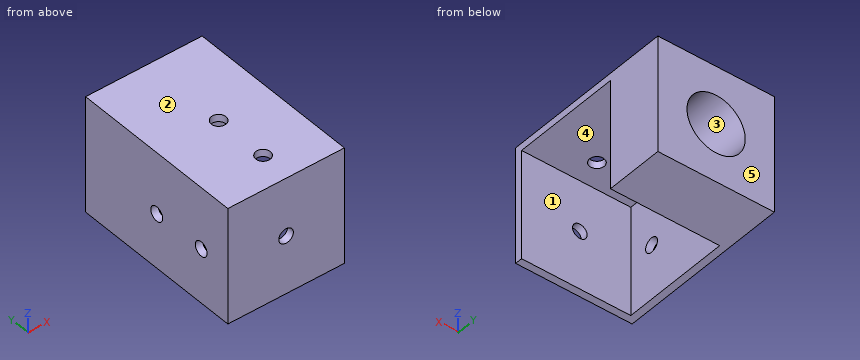
Autodesk Inventor part; units mm, degrees
ref_plane "YZ Plane" through (0, 0, 0) normal (1, 0, 0) x (0, 1, 0)
ref_plane "XZ Plane" through (0, 0, 0) normal (0, 1, 0) x (-1, 0, 0)
ref_plane "XY Plane" through (0, 0, 0) normal (0, 0, 1) x (1, 0, 0)
sketch "Sketch1" plane through (0, 0, 0) normal (0, 1, 0) x (-1, 0, 0)
  line L0 (0, 0) -> (50.8, 0)
  line L1 (50.8, 0) -> (50.8, -50.8)
  line L2 (50.8, -50.8) -> (0, -50.8)
  line L3 (0, -50.8) -> (0, 0)
  line L4 (47.625, -3.175) -> (3.175, -3.175)
  line L5 (3.175, -3.175) -> (3.175, -47.625)
  line L6 (3.175, -47.625) -> (47.625, -47.625)
  line L7 (47.625, -47.625) -> (47.625, -3.175)
  line L8 (47.625, -47.625) -> (47.625, -50.8)
  line L9 (3.175, -3.175) -> (0, -3.175)
  dimension "d0" = 50.8
  dimension "d1" = 50.8
  dimension "d2" = 3.175
extrude "Extrusion1" add sketch "Sketch1" against normal blind 25.4 contours L0 L1 L2 L8 L7 L4 L9 L3
sketch "Sketch2" plane through (0, 0, 0) normal (0, 1, 0) x (1, 0, 0)
  line L0 (-50.8, 0) -> (-50.8, 50.8)
  line L1 (-50.8, 0) -> (0, 0)
  line L2 (0, 0) -> (0, 50.8)
  line L3 (0, 50.8) -> (-50.8, 50.8)
  line L4 (-50.8, 50.8) -> (-50.8, 0)
  dimension "d5" = 50.8
extrude "Extrusion2" add sketch "Sketch2" along normal blind 25.4
sketch "Sketch3" plane through (0, 25.4, 0) normal (0, 1, 0) x (1, 0, 0)
  line L0 (-50.8, 0) -> (-50.8, 50.8) construction
  line L1 (-50.8, 0) -> (0, 50.8) construction
  line L2 (0, 0) -> (-50.8, 0) construction
  line L3 (0, 0) -> (-50.8, 50.8) construction
  point P0 (-25.61, 25.3161)
sketch "Sketch4" plane through (0, 25.4, 0) normal (0, 1, 0) x (1, 0, 0)
  point P0 (0, 0)
  point P1 (-25.3999, 25.4)
hole "Hole1" at (-25.3999, 25.4, -25.4) direction (0, -1, 0) diameter 25.4 end through all
sketch "Sketch5" plane through (0, -25.4, -3.175) normal (0, 0, -1) x (-1, 0, 0)
  line L0 (0, 25.4) -> (0, 0) construction
  line L1 (47.625, 0) -> (0, 0) construction
  line L2 (0, 25.4) -> (47.625, 0) construction
  line L3 (0, 25.4) -> (47.625, 25.4) construction
  line L4 (0, 0) -> (47.625, 25.4) construction
sketch "Sketch6" plane through (0, -25.4, -3.175) normal (0, 0, -1) x (-1, 0, 0)
  point P0 (0, 25.4)
  point P1 (23.8125, 12.7)
hole "Hole2" at (-23.8125, -12.7, -3.175) direction (0, 0, 1) diameter 6.35 end through all
sketch "Sketch7" plane through (-47.625, -25.4, -3.175) normal (1, 0, 0) x (0, 0, -1)
  line L0 (47.625, 0) -> (0, 0) construction
  line L1 (0, 25.4) -> (0, 0) construction
  line L2 (47.625, 0) -> (0, 25.4) construction
  line L3 (47.625, 25.4) -> (47.625, 0) construction
  line L4 (0, 0) -> (47.625, 25.4) construction
  point P0 (-3.175, 25.4)
sketch "Sketch8" plane through (-47.625, -25.4, -3.175) normal (1, 0, 0) x (0, 0, -1)
  point P0 (-3.175, 25.4)
  point P1 (23.8116, 12.6997)
hole "Hole3" at (-47.625, -12.7003, -26.9866) direction (-1, 0, 0) diameter 6.35 end through all
sketch "Sketch9" plane through (0, -25.4, 0) normal (0, -1, 0) x (1, 0, 0)
  line L0 (-50.8, -50.8) -> (-50.8, 0)
  line L1 (0, 0) -> (-50.8, 0)
  line L2 (-50.8, 0) -> (-50.8, -50.8)
  line L3 (-50.8, -50.8) -> (0, -50.8)
  line L4 (0, -50.8) -> (0, 0)
  line L5 (-47.625, -3.175) -> (-3.175, -3.175)
  line L6 (-3.175, -3.175) -> (-3.175, -47.625)
  line L7 (-3.175, -47.625) -> (-47.625, -47.625)
  line L8 (-47.625, -47.625) -> (-47.625, -3.175)
  line L9 (0, -3.175) -> (-47.625, -3.175)
  line L10 (-3.175, -3.175) -> (0, -3.175)
  line L11 (-47.625, -47.625) -> (-47.625, -50.8)
  point P0 (-3.175, -3.175)
extrude "Extrusion3" add sketch "Sketch9" along normal blind 25.4 contours L0 L1 L4 L9 L5 L8 L11 L3
sketch "Sketch10" plane through (0, -50.8, 0) normal (0, -1, 0) x (1, 0, 0)
  line L0 (0, 0) -> (-50.8, 0)
  line L1 (-50.8, 0) -> (-50.8, -50.8)
  line L2 (-50.8, -50.8) -> (0, -50.8)
  line L3 (0, -50.8) -> (0, 0)
extrude "Extrusion4" add sketch "Sketch10" against normal blind 3.175
sketch "Sketch11" plane through (0, 0, -3.175) normal (0, 0, -1) x (-1, 0, 0)
  line L0 (47.625, 0) -> (47.625, -47.625) construction
  line L1 (47.625, -47.625) -> (0, -25.4001) construction
  line L2 (0, 0) -> (0, -47.625) construction
  line L3 (0, -47.625) -> (47.625, -47.625) construction
  line L4 (47.625, -25.4001) -> (0, -47.625) construction
sketch "Sketch12" plane through (0, 0, -3.175) normal (0, 0, -1) x (-1, 0, 0)
  point P0 (0, 0)
  point P1 (23.8112, -36.5118)
hole "Hole4" at (-23.8112, -36.5118, -3.175) direction (0, 0, 1) diameter 6.35 end through all
sketch "Sketch13" plane through (-47.625, 0, -3.175) normal (1, 0, 0) x (0, 0, -1)
  line L0 (0, 0) -> (0, -47.625) construction
  line L1 (0, -47.625) -> (47.625, -47.625) construction
  line L2 (0, -25.4031) -> (47.625, -47.625) construction
  line L3 (0, -47.625) -> (47.625, -25.4031) construction
  line L4 (47.625, 0) -> (47.625, -47.625) construction
  point P0 (-3.175, 0)
sketch "Sketch14" plane through (-47.625, 0, -3.175) normal (1, 0, 0) x (0, 0, -1)
  point P0 (-3.175, 0)
  point P1 (23.8113, -36.5122)
hole "Hole5" at (-47.625, -36.5122, -26.9863) direction (-1, 0, 0) diameter 6.35 end through all
sketch "Sketch15" plane through (0, -47.625, 0) normal (0, 1, 0) x (1, 0, 0)
  line L0 (-50.8, 0) -> (-50.8, 50.8) construction
  line L1 (0, 0) -> (-50.8, 50.8) construction
  line L2 (0, 0) -> (0, 50.8) construction
  line L3 (-50.8, 0) -> (0, 50.8) construction
sketch "Sketch16" plane through (0, -47.625, 0) normal (0, 1, 0) x (1, 0, 0)
  point P0 (0, 0)
  point P1 (-25.4077, 25.4046)
hole "Hole6" at (-25.4077, -47.625, -25.4046) direction (0, -1, 0) diameter 6.35 end through all
properties part number "Bearing Housing"
The model under review builds one solid part; all positions refer to its coordinate system, in mm. Face numbers are marked on the shaded views. A direction names the side the tool comes from. Round coordinates to 2 decimals unless told otherwise and drop trailing zeros. Order: outer loops, then holes, each group sorted by start corner. A loop starts at its lowest first (then second) coordinate and runs counter-clockwise, first axis right, second up. Notation, with made-up numbers: M 50.5,69 L 68.5,69 A33 ccw 68.5,108 Z; hole C 58.5,-18.5 d10. An arc over 180 degrees is marked long. Use a Markdown table: item, result.
1) Consider section A-A (z = -27). Write out the cut boundary in (x, y) (3 decimals).
Report:
| item | result |
|---|---|
| outline | M -50.8,-50.8 L -28.153,-50.8 L -28.153,-47.625 L -47.625,-47.625 L -47.625,-39.687 L -50.8,-39.687 Z; M -50.8,-33.337 L -47.625,-33.337 L -47.625,-15.875 L -50.8,-15.875 Z; M -50.8,-9.525 L -47.625,-9.525 L -47.625,0 L -37.999,0 L -37.999,25.4 L -50.8,25.4 Z; M -22.663,-50.8 L 0,-50.8 L 0,-47.625 L -22.663,-47.625 Z; M -12.801,0 L 0,0 L 0,25.4 L -12.801,25.4 Z |
2) Consider section C-C (y = -11). Write out the cut boundary in (x, z) (3 decimals).
Report:
| item | result |
|---|---|
| outline | M -50.8,-50.8 L -47.625,-50.8 L -47.625,-29.668 L -50.8,-29.668 Z; M -50.8,-24.305 L -47.625,-24.305 L -47.625,-3.175 L -26.494,-3.175 L -26.494,0 L -50.8,0 Z; M -21.131,-3.175 L 0,-3.175 L 0,0 L -21.131,0 Z |
3) Wall thickness on line 1 along Y through (x, z) = (-30, -7) (3 decimals); line 2 along Z through (x, y) = (-26, 15.5); line 3 along Z through (x, y) = (-2.5, -22) (3 decimals): over which ranges is each line inside the solid? List them lowest first. Write a range as [from, to].
Report:
| item | result |
|---|---|
| line 1 | [-50.8, -47.625], [0, 25.4] |
| line 2 | [-50.8, -38.09], [-12.71, 0] |
| line 3 | [-3.175, 0] |
4) Consider section D-D (x = -34.5). Write out the cut boundary in (y, z) (3 decimals), then the cut area to 3 significant figures.
Report:
| item | result |
|---|---|
| outline | M -50.8,-50.8 L -47.625,-50.8 L -47.625,-3.175 L 0,-3.175 L 0,-16.541 L 25.4,-16.541 L 25.4,0 L -50.8,0 Z; M 0,-50.8 L 25.4,-50.8 L 25.4,-34.259 L 0,-34.259 Z |
| area | 1,150 mm^2 |
5) Draft analysis for pull direction Z (two halves, no side actions). For the marked faces 1, 2 and 3, state which applies: released by +Z, released by -Z, zero draft, split by the parting line, or undercut.
Report:
| item | result |
|---|---|
| face 1 | zero draft |
| face 2 | released by +Z |
| face 3 | undercut |
6) Insertion check: pin 1 (1 mm diameter, centred on x = -9, y = -9.5, fed in from -Z) (3 decimals); pin 2 (4 mm diameter, centred on x = -25.41, z = -25.4, fed in from +Y). Each pin has a flat end and moves straight along its axis. Give the tip position at first contact, or say it passes through.
Report:
| item | result |
|---|---|
| pin 1 | z = -3.175 |
| pin 2 | through |
7) Tool access review of the marked faces 4 and 5: name each direction out of +Z, -Z, +X, -X, +Y, -Y from which nothing blocks a thin tool from reaching the whole face with its end or side.
Report:
| item | result |
|---|---|
| face 4 | -Z, +X |
| face 5 | +Z, -Z, +X, -X, +Y |
8) Consider section B-B (x = -46.5). Write out the cut boundary in (y, z) (3 decimals).
Report:
| item | result |
|---|---|
| outline | M -50.8,-50.8 L -47.625,-50.8 L -47.625,-3.175 L 0,-3.175 L 0,-50.8 L 25.4,-50.8 L 25.4,0 L -50.8,0 Z |
